Autodesk Fusion 360 part; units mm, degrees
sketch "Sketch1" plane through (0, 0, 0) normal (0, 0, 1) x (1, 0, 0) in component "base"
  circle A0 centre (43.9809, 31.3929) radius 50
  circle A1 centre (43.9809, 31.3929) radius 46
  circle A2 centre (43.9809, 31.3929) radius 19
  circle A3 centre (43.9809, 31.3929) radius 15
  dimension "d1" = 100
  dimension "d2" = 4
  dimension "d4" = 4
  dimension "d6" = 30
extrude "Extrude1" add sketch "Sketch1" against normal blind 20 contours A0 | A1 makes body 1 in component "base"
extrude "Extrude2" cut sketch "Sketch1" against normal blind 16 contours A1 bodies 1 in component "base"
extrude "Extrude3" add sketch "Sketch1" against normal blind 25 from surface at -16 contours A2 bodies 1 in component "base"
move_body "Move1" bodies 1 to x (1, 0, 0) y (0, -1, 0) z (0, 0, -1) at (0, -37.2143, -80) in component "base"
move_body "Move2" bodies 1 to x (1, 0, 0) y (0, 1, 0) z (0, 0, 1) at (0, 100, 80) in component "base"
copy_body "CutPasteBodies1" bodies 1 removing the originals makes body 2 in component "base"
component "base" placed x (1, 0, 0) y (0, 1, 0) z (0, 0, 1) at (0, 0, 0)
component "Component" placed x (1, 0, 0) y (0, 1, 0) z (0, 0, 1) at (0, 0, 0)
equation "d2 = wallthickness"
equation "wallthickness = 4 mm"
equation "d4 = wallthickness"
equation "motorDiameter = 30 mm"
equation "d6 = motorDiameter"
equation "baseHeight = 20 mm"
equation "motorBaseHeight = 25 mm"
equation "d11 = wallthickness - baseHeight"
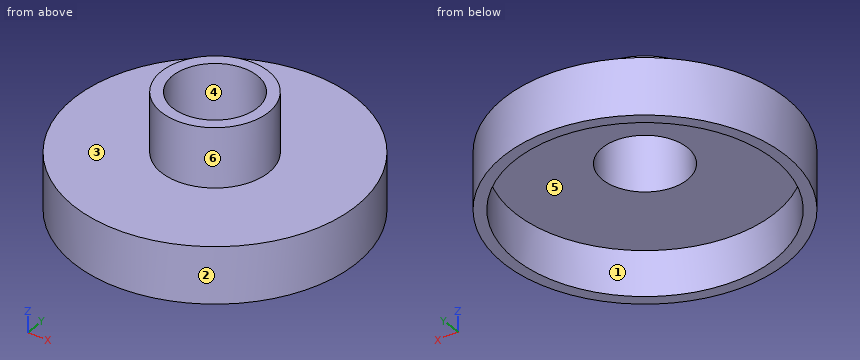
Work out the finished part from the listing and answer in its coordinate system (mm). Face numbers are marked on the shaded views. A direction names the side the tool comes from. Round coordinates to 2 decimals unless told otherwise and drop trailing zeros. Write each loop counter-clockwise with the first axis right and the second up, starting at its lowest first coordinate (ties: lowest second). Pieces come first, ordered by that corner, then holes.
1) Straight lines are drawn through the part: line 1 (Z direction, x = 49.5, y = 68); line 2 (X direction, y = 36, z = 24); line 3 (Z direction, x = 60.5, y = 40.5). For each, find the intervals that lie inside material, in ascending order.
2) Given pin 1 Ø6 at (x, y) = (70, 55.5) entering from +Z; pin 2 Ø1.5 at (y, z) = (19, 10) entering from -X; pin 3 Ø1 at (x, z) = (54.5, 5.5) entering from -Y, each flat-ended and moving along its own axis, determine where each tip first touches the part or whether it passes through.
3) The mould has two halves that part along Y. Classify the marked faces 1, 2 and 3: pulls with the +Y half, pulls with the -Y half, needs draft (parallel to the pull), parting line crosses it, or undercut.
4) A cutting plane is placed at D-D (y = -3.5). Give the vertices of the cut face in (x, z), plus the area to 3 significant figures.
5) A cutting plane is placed at A-A (y = 38). Give the vertices of the cut face in (x, z), plus the area to 3 significant figures.
6) A cutting plane is placed at B-B (x = 57.5). Give the vertices of the cut face in (y, z).
7) A tool of negligible diameter and unlimited length cuts with its end or side. For the marked faces 4, 5 and 6, from which of +Z, -Z, +X, -X, +Y, -Y can it reach the whole face along a straight path? Write none if from no direction.
8) A cutting plane is placed at C-C (x = 86). Give the vertices of the cut face in (y, z), plus the area to 3 significant figures.
Completed:
1. line 1: z = 16 to 20
1. line 2: x = 25.55 to 29.71, 58.26 to 62.41
1. line 3: z = 16 to 41
2. pin 1: stops at z = 20
2. pin 2: stops at x = -4.64
2. pin 3: stops at y = -17.59
3. face 1: undercut
3. face 2: parting line crosses it
3. face 3: needs draft
4. outline: (8.17, 0) - (14.01, 0) - (14.01, 16) - (73.96, 16) - (73.96, 0) - (79.79, 0) - (79.79, 20) - (8.17, 20) - close
4. area: 473 mm2
5. outline: (-5.58, 0) - (-1.54, 0) - (-1.54, 16) - (30.51, 16) - (30.51, 41) - (26.17, 41) - (26.17, 20) - (-5.58, 20) - close; (57.45, 16) - (89.5, 16) - (89.5, 0) - (93.54, 0) - (93.54, 20) - (61.8, 20) - (61.8, 41) - (57.45, 41) - close
5. area: 601 mm2
6. outline: (-16.74, 0) - (-12.58, 0) - (-12.58, 16) - (24.89, 16) - (24.89, 41) - (18.04, 41) - (18.04, 20) - (-16.74, 20) - close; (37.89, 16) - (75.36, 16) - (75.36, 0) - (79.53, 0) - (79.53, 20) - (44.74, 20) - (44.74, 41) - (37.89, 41) - close
7. face 4: +Z, -Z
7. face 5: -Z
7. face 6: +Z
8. outline: (4.29, 0) - (12.67, 0) - (12.67, 16) - (50.11, 16) - (50.11, 0) - (58.49, 0) - (58.49, 20) - (4.29, 20) - close
8. area: 485 mm2
